```python
from build123d import *

# Parameters (mm, degrees)
F0_W     = 36.9
F0_H     = 10
F0_W_2   = 10
F0_H_2   = 36.9
F1_DEPTH = 5
F2_DEPTH = 10
F3_SIZE  = 1


with BuildPart() as f1:
    # F0 (on Top) → F1 (new body)
    with BuildSketch(Plane.XY):
        Polygon((49.6, 12.7), (49.6, 5), (49.6, -5), (49.6, -12.7), (75, -12.7), (75, -5), (75, 5), (75, 12.7), align=None)
        with Locations((31.15, 0)):
            Rectangle(F0_W, F0_H)
        Polygon((5, 12.7), (-5, 12.7), (-12.7, 12.7), (-12.7, 5), (-12.7, -5), (-12.7, -12.7), (-5, -12.7), (5, -12.7), (12.7, -12.7), (12.7, -5), (12.7, 5), (12.7, 12.7), align=None)
        with Locations((0, -31.15)):
            Rectangle(F0_W_2, F0_H_2)
        Polygon((5, -49.6), (-5, -49.6), (-12.7, -49.6), (-12.7, -75), (-5, -75), (5, -75), (12.7, -75), (12.7, -49.6), align=None)
        with Locations((-31.15, 0)):
            Rectangle(F0_W, F0_H)
        Polygon((-49.6, -5), (-49.6, 5), (-49.6, 12.7), (-75, 12.7), (-75, 5), (-75, -5), (-75, -12.7), (-49.6, -12.7), align=None)
        with Locations((0, 31.15)):
            Rectangle(F0_W_2, F0_H_2)
        Polygon((-5, 75), (-12.7, 75), (-12.7, 49.6), (-5, 49.6), (5, 49.6), (12.7, 49.6), (12.7, 75), (5, 75), align=None)
    extrude(amount=F1_DEPTH)

    # F0 (on Top) → F2 (join)
    with BuildSketch(Plane.XY):
        Polygon((-49.6, -5), (-49.6, 5), (-49.6, 12.7), (-75, 12.7), (-75, 5), (-75, -5), (-75, -12.7), (-49.6, -12.7), align=None)
        Polygon((-5, 75), (-12.7, 75), (-12.7, 49.6), (-5, 49.6), (5, 49.6), (12.7, 49.6), (12.7, 75), (5, 75), align=None)
        Polygon((49.6, 12.7), (49.6, 5), (49.6, -5), (49.6, -12.7), (75, -12.7), (75, -5), (75, 5), (75, 12.7), align=None)
        Polygon((5, 12.7), (-5, 12.7), (-12.7, 12.7), (-12.7, 5), (-12.7, -5), (-12.7, -12.7), (-5, -12.7), (5, -12.7), (12.7, -12.7), (12.7, -5), (12.7, 5), (12.7, 12.7), align=None)
        Polygon((5, -49.6), (-5, -49.6), (-12.7, -49.6), (-12.7, -75), (-5, -75), (5, -75), (12.7, -75), (12.7, -49.6), align=None)
    extrude(amount=F2_DEPTH)

    # F3
    f3_edges = [f1.edges().sort_by_distance(p)[0] for p in [
        (0, 75, 0),
        (-12.7, 62.3, 0),
        (-8.85, 49.6, 0),
        (-5, 31.15, 0),
        (-8.85, 12.7, 0),
        (-12.7, 8.85, 0),
        (-31.15, 5, 0),
        (-49.6, 8.85, 0),
        (-62.3, 12.7, 0),
        (-75, 0, 0),
        (-62.3, -12.7, 0),
        (-49.6, -8.85, 0),
        (-31.15, -5, 0),
        (-12.7, -8.85, 0),
        (-8.85, -12.7, 0),
        (-5, -31.15, 0),
        (-8.85, -49.6, 0),
        (-12.7, -62.3, 0),
        (0, -75, 0),
        (12.7, -62.3, 0),
        (8.85, -49.6, 0),
        (5, -31.15, 0),
        (8.85, -12.7, 0),
        (12.7, -8.85, 0),
        (31.15, -5, 0),
        (49.6, -8.85, 0),
        (62.3, -12.7, 0),
        (75, 0, 0),
        (62.3, 12.7, 0),
        (49.6, 8.85, 0),
        (31.15, 5, 0),
        (12.7, 8.85, 0),
        (8.85, 12.7, 0),
        (5, 31.15, 0),
        (8.85, 49.6, 0),
        (12.7, 62.3, 0),
    ]]
    chamfer(f3_edges, length=F3_SIZE)


solid = f1.part
```
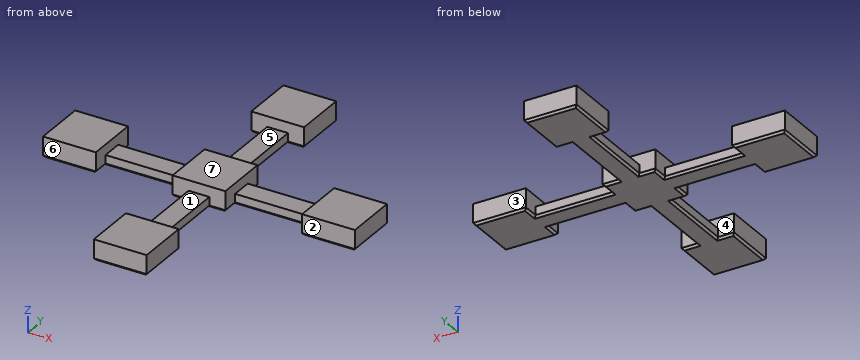
Part model, mm, in its own coordinate system. Face numbers are marked on the shaded views. A direction names the side the tool comes from. Round coordinates to 2 decimals unless told otherwise and drop trailing zeros. Write each loop counter-clockwise with the first axis right and the second up, starting at its lowest first coordinate (ties: lowest second). Pieces come first, ordered by that corner, then holes. Notation, with made-up numbers: M 72.5,-26.75 L 104.5,-26.75 A34 ccw 104.5,7.25 Z; hole C -27,-22.5 d3. An arc over 180 degrees is marked long. One line per question, with ' | ' between items.
(1) 3-axis set-ups, long thin cutter, end or side, ignore diameter. For the marked faces 1, 2, 3 and 4: which of +Z, -Z, +X, -X, +Y, -Y reach the whole face in a straight line?
Answer key:
face 1: +Z, +X, -X | face 2: +Z, -Z, +X, -Y | face 3: +Z, -Z, +X, +Y | face 4: +Z
(2) Saw through at B-B on x = 54. Write the cut outline in (y, z).
Answer key:
outline: M -12.7,1 L -11.7,0 L 11.7,0 L 12.7,1 L 12.7,10 L -12.7,10 Z
(3) Saw through at C-C on y = 22. Write the cut outline in (x, z), then the cut area to 3 significant figures.
Answer key:
outline: M -5,1 L -4,0 L 4,0 L 5,1 L 5,5 L -5,5 Z | area: 49.0 mm^2
(4) Probe line 1 along Y through (x, z) = (11.5, 4); line 2 along X through (y, z) = (64, 5.5); line 3 along Y through (x, z) = (-37.5, 1). List the from-to ranges inside material, lowest first.
Answer key:
line 1: y = -75 to -49.6, -12.7 to 12.7, 49.6 to 75 | line 2: x = -12.7 to 12.7 | line 3: y = -5 to 5
(5) Pin check, flat tips, straight feed: pin 1 (4.5 mm diameter, centred on y = 66.5, z = 7, fed in from -X); pin 2 (3 mm diameter, centred on x = 26.5, y = 0.5, fed in from +Z); pin 3 (1.2 mm diameter, centred on x = -34, z = 2.5, fed in from +Y). Stop position of each tip, or through.
Answer key:
pin 1: stops at x = -12.7 | pin 2: stops at z = 5 | pin 3: stops at y = 5
(6) Saw through at A-A on z = 7.25. Write the cut outline in (x, y).
Answer key:
outline: M -75,-12.7 L -49.6,-12.7 L -49.6,12.7 L -75,12.7 Z; M -12.7,-75 L 12.7,-75 L 12.7,-49.6 L -12.7,-49.6 Z; M -12.7,-12.7 L 12.7,-12.7 L 12.7,12.7 L -12.7,12.7 Z; M -12.7,49.6 L 12.7,49.6 L 12.7,75 L -12.7,75 Z; M 49.6,-12.7 L 75,-12.7 L 75,12.7 L 49.6,12.7 Z
(7) Two-plate mould, pull along Y, no slides. Class the marked faces 5, 6 and 7: released by +Y, released by -Y, zero draft, split by the parting line, or undercut.
Answer key:
face 5: undercut | face 6: released by -Y | face 7: zero draft
